from build123d import *

# Parameters (mm, degrees)
SKETCH1_R                = 4
BOSS_EXTRUDE1_DEPTH      = 2
SKETCH2_R                = 10
SKETCH2_R_2              = 3.8
BOSS_EXTRUDE2_DEPTH      = 2
SKETCH4_W                = 12
SKETCH4_H                = 0.2
CUT_EXTRUDE1_DEPTH       = 4
FILLET3_R                = 0.35
FILLET4_R                = 0.15
FILLET6_R                = 2
SKETCH13_R               = 5.25
CUT_EXTRUDE5_DEPTH       = 1.25
REVOLVE2_ANGLE           = 30
CIRPATTERN2_COUNT        = 3
CHAMFER1_SIZE            = 0.5
CHAMFER1_SIZE2           = 0.181985117
FILLET14_R               = 0.25
BOSS_EXTRUDE8_START      = -0.75
BOSS_EXTRUDE8_DEPTH      = 2
BOSS_EXTRUDE8_DRAFT      = -3
SKETCH16_W               = 2
SKETCH16_H               = 1.934959958
BOSS_EXTRUDE9_DEPTH      = 1.25
BOSS_EXTRUDE9_TAPER      = 3
CIRPATTERN3_COUNT        = 3
CIRPATTERN3_START        = -0.75
CIRPATTERN3_COPY_1_DEPTH = 2
CIRPATTERN3_COPY_1_DRAFT = -3
CIRPATTERN3_COPY_2_DEPTH = 2
CIRPATTERN3_COPY_2_DRAFT = -3


with BuildPart() as part:
    # Sketch1 → Boss-Extrude1 (new body)
    with BuildSketch(Plane(origin=(0, 0, 0), x_dir=(1, 0, 0), z_dir=(0, 1, 0))):
        Polygon((-6, 6), (-6, -13.291502622), (-6, -19), (-2.70227506, -19), (-3.619175359, -13.8), (0, -13.8), (3.619175359, -13.8), (2.70227506, -19), (6, -19), (6, -13.291502622), (6, 6), align=None)
        with Locations(Location((0, 0, 0), (0, 0, 270))):
            Circle(SKETCH1_R, mode=Mode.SUBTRACT)
    extrude(amount=BOSS_EXTRUDE1_DEPTH)

    # Sketch2 → Boss-Extrude2 (add)
    with BuildSketch(Plane(origin=(0, 0, 0), x_dir=(1, 0, 0), z_dir=(0, 1, 0))):
        Circle(SKETCH2_R)
        with Locations(Location((0, 0, 0), (0, 0, 270))):
            Circle(SKETCH2_R_2, mode=Mode.SUBTRACT)
    extrude(amount=BOSS_EXTRUDE2_DEPTH)

    # Sketch4 → Cut-Extrude1 (cut)
    with BuildSketch(Plane(origin=(0, 2, 0), x_dir=(1, 0, 0), z_dir=(0, 1, 0))):
        with Locations((0, -18.9)):
            Rectangle(SKETCH4_W, SKETCH4_H)
    extrude(amount=-CUT_EXTRUDE1_DEPTH, mode=Mode.SUBTRACT)

    # Fillet3
    fillet3_edges = [part.edges().sort_by_distance(p)[0] for p in [
        (3.619175359, 1, 13.8),
        (-3.619175359, 1, 13.8),
    ]]
    fillet(fillet3_edges, radius=FILLET3_R)

    # Fillet4
    fillet4_edges = [part.edges().sort_by_distance(p)[0] for p in [
        (2.737540456, 1, 18.8),
        (-2.737540456, 1, 18.8),
    ]]
    fillet(fillet4_edges, radius=FILLET4_R)

    # Fillet6
    fillet6_edges = [part.edges().sort_by_distance(p)[0] for p in [
        (6, 1, 8),
        (-6, 1, 8),
    ]]
    fillet(fillet6_edges, radius=FILLET6_R)

    # Sketch13 → Cut-Extrude5 (cut)
    with BuildSketch(Plane(origin=(0, 2, 0), x_dir=(1, 0, 0), z_dir=(0, 1, 0))):
        with Locations(Location((0, 0, 0), (0, 0, 270))):
            Circle(SKETCH13_R)
    extrude(amount=-CUT_EXTRUDE5_DEPTH, mode=Mode.SUBTRACT)

    # Sketch12 → Revolve2 (revolve, symmetric)
    with BuildSketch(Plane(origin=(0, 0, 0), x_dir=(0, 0, -1), z_dir=(1, 0, 0))) as revolve2_sk:
        Polygon((-4, 0), (-3.4, 2), (-4.4, 2), (-5, 0), align=None)
    revolve2 = revolve(axis=Axis((0, 0, 0), (0, 1, 0)), revolution_arc=REVOLVE2_ANGLE / 2)
    revolve2 = revolve2 + revolve(revolve2_sk.sketch, axis=Axis((0, 0, 0), (0, -1, 0)), revolution_arc=REVOLVE2_ANGLE / 2)

    # CirPattern2: Revolve2 ×3 about axis
    cirpattern2_axis = Axis((0, 0, 0), (0, 1, 0))
    for i in range(1, CIRPATTERN2_COUNT):
        add(revolve2.rotate(cirpattern2_axis, i * 360 / CIRPATTERN2_COUNT))

    # Chamfer1
    chamfer1_edges = [part.edges().sort_by_distance(p)[0] for p in [
        (0, 0, -3.8),
    ]]
    chamfer1_side = [part.faces().sort_by_distance(p)[0] for p in [
        (0, 0.375, -3.8),
    ]]
    chamfer(chamfer1_edges, length=CHAMFER1_SIZE, length2=CHAMFER1_SIZE2, reference=chamfer1_side[0])

    # Fillet14
    fillet14_edges = [part.edges().sort_by_distance(p)[0] for p in [
        (0, 0.75, -5.25),
        (0, 0.75, 4.775),
        (-4.135271303, 0.75, -2.3875),
        (4.135271303, 0.75, -2.3875),
    ]]
    fillet(fillet14_edges, radius=FILLET14_R)


with BuildPart() as boss_extrude8_tool:
    # Sketch15 → Boss-Extrude8 (with draft: the straight prism first)
    with BuildSketch(Plane.XZ.offset(BOSS_EXTRUDE8_START)):
        with BuildLine():
            Line((1, -4.898979486), (1, -3.666060556))
            ThreePointArc((1, -3.666060556), (0, -3.8), (-1, -3.666060556))
            Line((-1, -3.666060556), (-1, -4.898979486))
            ThreePointArc((-1, -4.898979486), (0, -5), (1, -4.898979486))
        make_face()
    extrude(amount=-BOSS_EXTRUDE8_DEPTH)
    # Boss-Extrude8: the draft: its side faces are tilted about the plane it starts from
    boss_extrude8_sides = [boss_extrude8_tool.faces().sort_by_distance(p)[0] for p in [
        (1, 1.75, -4.282520021),
        (0, 1.75, -3.8),
        (-1, 1.75, -4.282520021),
        (0, 1.75, -5),
    ]]
    draft(boss_extrude8_sides, Plane.XZ.offset(BOSS_EXTRUDE8_START), BOSS_EXTRUDE8_DRAFT)


with BuildPart() as part_1:
    add(part.part)

    # Boss-Extrude8: add boss_extrude8_tool
    add(boss_extrude8_tool.part)

    # Sketch16 → Boss-Extrude9 (add)
    with BuildSketch(Plane(origin=(0, 0.75, 0), x_dir=(1, 0, 0), z_dir=(0, 1, 0))):
        with Locations((0, 5.25)):
            Rectangle(SKETCH16_W, SKETCH16_H)
    boss_extrude9 = extrude(amount=BOSS_EXTRUDE9_DEPTH, taper=BOSS_EXTRUDE9_TAPER)

    # CirPattern3: Boss-Extrude9 ×3 about axis
    cirpattern3_axis = Axis((0, 0, 0), (0, 1, 0))
    for i in range(1, CIRPATTERN3_COUNT):
        add(boss_extrude9.rotate(cirpattern3_axis, i * 360 / CIRPATTERN3_COUNT))


with BuildPart() as cirpattern3_copy_1_tool:
    # CirPattern3 copy 1 sketch → CirPattern3 copy 1 (with draft: the straight prism first)
    with BuildSketch(Plane(origin=(0, 0, 0), x_dir=(-0.4999999999999998, 0, -0.8660254037844387), z_dir=(0, -1, 0)).offset(CIRPATTERN3_START)):
        with BuildLine():
            Line((1, -4.898979486), (1, -3.666060556))
            ThreePointArc((1, -3.666060556), (0, -3.8), (-1, -3.666060556))
            Line((-1, -3.666060556), (-1, -4.898979486))
            ThreePointArc((-1, -4.898979486), (0, -5), (1, -4.898979486))
        make_face()
    extrude(amount=-CIRPATTERN3_COPY_1_DEPTH)
    # CirPattern3 copy 1: the draft: its side faces are tilted about the plane it starts from
    cirpattern3_copy_1_sides = [cirpattern3_copy_1_tool.faces().sort_by_distance(p)[0] for p in [
        (-4.20877113, 1.75, 1.275234607),
        (-3.290896534, 1.75, 1.9),
        (-3.20877113, 1.75, 3.007285414),
        (-4.330127019, 1.75, 2.5),
    ]]
    draft(cirpattern3_copy_1_sides, Plane(origin=(0, 0, 0), x_dir=(-0.4999999999999998, 0, -0.8660254037844387), z_dir=(0, -1, 0)).offset(CIRPATTERN3_START), CIRPATTERN3_COPY_1_DRAFT)


with BuildPart() as part_2:
    add(part_1.part)

    # CirPattern3 copy 1: add cirpattern3_copy_1_tool
    add(cirpattern3_copy_1_tool.part)


with BuildPart() as cirpattern3_copy_2_tool:
    # CirPattern3 copy 2 sketch → CirPattern3 copy 2 (with draft: the straight prism first)
    with BuildSketch(Plane(origin=(0, 0, 0), x_dir=(-0.5000000000000004, 0, 0.8660254037844384), z_dir=(0, -1, 0)).offset(CIRPATTERN3_START)):
        with BuildLine():
            Line((1, -4.898979486), (1, -3.666060556))
            ThreePointArc((1, -3.666060556), (0, -3.8), (-1, -3.666060556))
            Line((-1, -3.666060556), (-1, -4.898979486))
            ThreePointArc((-1, -4.898979486), (0, -5), (1, -4.898979486))
        make_face()
    extrude(amount=-CIRPATTERN3_COPY_2_DEPTH)
    # CirPattern3 copy 2: the draft: its side faces are tilted about the plane it starts from
    cirpattern3_copy_2_sides = [cirpattern3_copy_2_tool.faces().sort_by_distance(p)[0] for p in [
        (3.20877113, 1.75, 3.007285414),
        (3.290896534, 1.75, 1.9),
        (4.20877113, 1.75, 1.275234607),
        (4.330127019, 1.75, 2.5),
    ]]
    draft(cirpattern3_copy_2_sides, Plane(origin=(0, 0, 0), x_dir=(-0.5000000000000004, 0, 0.8660254037844384), z_dir=(0, -1, 0)).offset(CIRPATTERN3_START), CIRPATTERN3_COPY_2_DRAFT)


with BuildPart() as part_3:
    add(part_2.part)

    # CirPattern3 copy 2: add cirpattern3_copy_2_tool
    add(cirpattern3_copy_2_tool.part)


solid = part_3.part
Here's how the part is built. I have some questions about the finished solid (model axes, mm). A direction names the side the tool comes from. Give positions to 0.01 mm unless a question says otherwise; leave off trailing zeros. Order: outer loops, then holes, each group sorted by start corner. A loop starts at its lowest first (then second) coordinate and runs counter-clockwise, first axis right, second up. Notation, with made-up numbers: M 63,22.25 L 71,22.25 A16 cw 71,39.25 Z; hole C 77.5,-8.5 d10. An arc over 180 degrees is marked long. Answer as a JSON object with one key per item and string values. Group by question number.
1) Please list where these lines run through material, in increasing order: L1, parallel to Z at x = 0.5, y = 1.4; L2, parallel to X at y = 0.7, z = 0; L3, parallel to Z at x = 0, y = 0.65. Write a range as [from, to].
2) I'm going to push flat-ended pins straight in: pin 1 Ø0.6 at (x, z) = (-3, -2) entering from +Y; pin 2 Ø0.6 at (x, y) = (0.5, 1) entering from +Z; pin 3 Ø0.6 at (y, z) = (1, 12.5) entering from -X. Where does each tip first touch, or does it pass through?
3) On a 3-axis mill with a long thin cutter (end or side, diameter ignored), from which of +Z, -Z, +X, -X, +Y, -Y can I reach the whole of each face in a straight line? I mean faces 5 (the conical face through (0.01, 1.34, 3.6)), 6 (the flat face through (1.4, 0.75, 3.9)), 7 (the flat face through (-4, 2.75, 2)), 8 (the flat face through (3, 2, -2)). Say none if no direction works.
4) Suppose I cut it at C-C, the plane y = 1.7. Count the separate pieces of the cut face and the enclosed holes in it, plus the area to 3 significant figures.
5) Suppose I cut it at D-D, the plane z = 13. Write out the boundary of the cut face in (x, y), plus the area to 3 significant figures.
6) Suppose I cut it at A-A, the plane z = 0. Write out the boundary of the cut face in (x, y), plus the area to 3 significant figures.
7) We'd pull the mould along X, two halves only. Please class faces 1 (the flat face through (6, 1, 14)), 2 (the flat face through (-3.36, 1.764, 3.033)), 3 (the flat face through (-6, 1, 14)), 4 (the flat face through (-4, 1, 18.8)): pulls with the +X half, pulls with the -X half, needs draft (parallel to the pull), parting line crosses it, or undercut.
Results found:
{
 "1": {"L1": "[-9.99, -3.8], [3.54, 4.55], [5.23, 13.8]", "L2": "[-10, -3.8], [3.8, 10]", "L3": "[-10, -3.8], [3.8, 13.8]"},
 "2": {"pin 1": "y = 2", "pin 2": "z = 13.8", "pin 3": "x = -6"},
 "3": {"face 5": "-Y", "face 6": "+Y", "face 7": "+Z, -Z, +X, -X, +Y", "face 8": "-Z, +X, -X, +Y"},
 "4": {"separate pieces": "4", "enclosed holes": "1", "area": "324 mm²"},
 "5": {"outline": "M -6,0 L 6,0 L 6,2 L -6,2 Z", "area": "24.0 mm²"},
 "6": {"outline": "M -10,0 L -3.98,0 L -3.8,0.5 L -3.8,0.75 L -5,0.75 A0.25 cw -5.25,1 L -5.25,2 L -10,2 Z; M 3.8,0.5 L 3.98,0 L 10,0 L 10,2 L 5.25,2 L 5.25,1 A0.25 cw 5,0.75 L 3.8,0.75 Z", "area": "21.1 mm²"},
 "7": {"face 1": "pulls with the +X half", "face 2": "undercut", "face 3": "pulls with the -X half", "face 4": "needs draft"}
}
